Study the drawing (mm; zero at the part's minimum x, y, z) and answer. Coordinates: 2 decimals unless noted, no trailing zeros. Order: outer loops, then holes, each group sorted by start corner. A loop starts at its lowest first (then second) coordinate and runs counter-clockwise, first axis right, second up. Notation, with made-up numbers: M 21,43 L 67,43 A31 cw 67,81 Z; hole C -39.5,-39 d9. An arc over 180 degrees is marked long. One line per item, written item: value. Start each with the question number.
Q1. Straight lines are drawn through the part: line 1 along Y through (x, z) = (9.5, 0.9); line 2 along Z through (x, y) = (21, 13.5). For each, find the intervals that lie inside material, in ascending order. Write a range as [from, to].
Q2. The part is cut by section A-A on z = 0.8. Give the vertices of the cut face in (x, y).
Q3. This flat-tipped pin is pushed along its axis until it touches: pin 1 Ø2 at (x, y) = (15.5, 18) entering from -Z. Where does it stop, or does it pass through?
Q4. The part is cut by section B-B on y = 17. Give the vertices of the cut face in (x, z), then the cut area to 3 significant figures.
Q5. Determine the mould class of the marked faces 1 and 2 for opening direction Y: pulls with the +Y half, pulls with the -Y half, needs draft (parallel to the pull), parting line crosses it, or undercut.
Q6. The part is cut by section D-D on x = 24.5. Give the vertices of the cut face in (y, z).
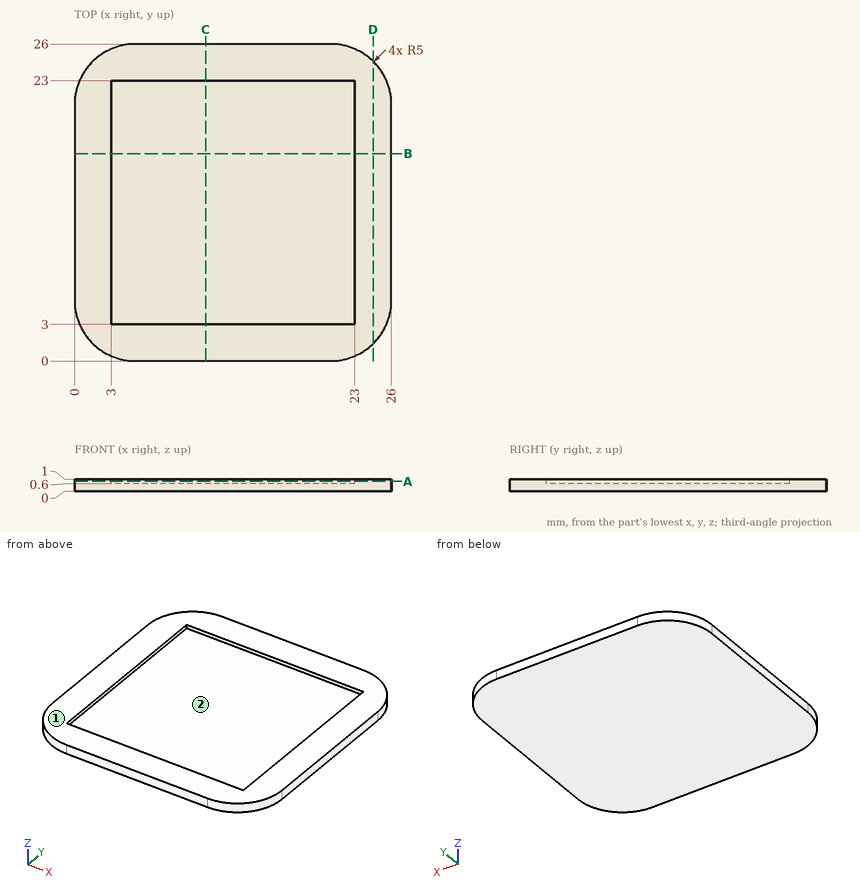
Output:
1. line 1: y = [0, 3], [23, 26]
1. line 2: z = [0, 0.6]
2. outline: M 0,5 A5 ccw 5,0 L 21,0 A5 ccw 26,5 L 26,21 A5 ccw 21,26 L 5,26 A5 ccw 0,21 Z; hole M 3,3 L 23,3 L 23,23 L 3,23 Z
3. pin 1: stops at z = 0
4. outline: M 0,0 L 26,0 L 26,1 L 23,1 L 23,0.6 L 3,0.6 L 3,1 L 0,1 Z
4. area: 18.0 mm^2
5. face 1: needs draft
5. face 2: undercut
6. outline: M 1.43,0 L 24.57,0 L 24.57,1 L 1.43,1 Z
